from build123d import *
from build123d.topology import SkipClean

# Parameters (mm, degrees)
SKETCH2_R               = 69.85
BOSS_EXTRUDE1_DEPTH     = 4.233333
BOSS_EXTRUDE2_DEPTH     = 38.1
FILLET3_R               = 12.7
FILLET4_R               = 12.7
FILLET5_R               = 12.7
BOSS_EXTRUDE3_DEPTH     = 38.1
CUT_EXTRUDE1_DEPTH      = 108.471653
CUT_EXTRUDE1_DEPTH_BACK = 108.471653
SKETCH5_R               = 4.5085
FILLET6_R               = 12.7


with BuildPart() as part:
    # Sketch2 → Boss-Extrude1 (new body)
    with BuildSketch(Plane(origin=(0, 0, 0), x_dir=(1, 0, 0), z_dir=(0, 1, 0))):
        with Locations(Location((0, 0, 0), (0, 0, 270))):
            Circle(SKETCH2_R)
    extrude(amount=BOSS_EXTRUDE1_DEPTH)

    # Sketch3 → Boss-Extrude2 (add)
    with BuildSketch(Plane(origin=(0, 4.233333, 0), x_dir=(1, 0, 0), z_dir=(0, 1, 0))):
        with BuildLine():
            Line((-16.709043, -54.652817), (-20.422164, -66.797887))
            ThreePointArc((-20.422164, -66.797887), (0, -69.85), (20.422164, -66.797887))
            Line((20.422164, -66.797887), (16.709043, -54.652817))
            ThreePointArc((16.709043, -54.652817), (0, -57.15), (-16.709043, -54.652817))
        make_face()
        with BuildLine():
            ThreePointArc((20.422164, 66.797887), (0, 69.85), (-20.422164, 66.797887))
            Line((-20.422164, 66.797887), (-16.709043, 54.652817))
            ThreePointArc((-16.709043, 54.652817), (0, 57.15), (16.709043, 54.652817))
            Line((16.709043, 54.652817), (20.422164, 66.797887))
        make_face()
    extrude(amount=BOSS_EXTRUDE2_DEPTH)

    # Fillet3
    fillet3_edges = [part.edges().sort_by_distance(p)[0] for p in [
        (-16.709043, 23.283333, -54.652817),
    ]]
    fillet(fillet3_edges, radius=FILLET3_R)

    # Fillet4
    fillet4_edges = [part.edges().sort_by_distance(p)[0] for p in [
        (16.709043, 23.283333, 54.652817),
    ]]
    fillet(fillet4_edges, radius=FILLET4_R)

    # Fillet5
    fillet5_edges = [part.edges().sort_by_distance(p)[0] for p in [
        (-16.709043, 23.283333, 54.652817),
    ]]
    fillet(fillet5_edges, radius=FILLET5_R)

    # Sketch4 → Boss-Extrude3 (add)
    with SkipClean():  # the faces are left unmerged after this step: merging them gives an invalid solid
        with BuildSketch(Plane(origin=(0, 4.233333, 0), x_dir=(1, 0, 0), z_dir=(0, 1, 0))):
            with BuildLine():
                Line((59.670481, 21.718279), (65.63753, 23.890107))
                ThreePointArc((65.63753, 23.890107), (69.85, 0), (65.63753, -23.890107))
                Line((65.63753, -23.890107), (59.670481, -21.718279))
                ThreePointArc((59.670481, -21.718279), (63.5, 0), (59.670481, 21.718279))
            make_face()
        extrude(amount=BOSS_EXTRUDE3_DEPTH)

    # Sketch5 → Cut-Extrude1 (cut, two sides: drawn at the far end of the back side and taken through both)
    with SkipClean():  # the faces are left unmerged after this step: merging them gives an invalid solid
        with BuildSketch(Plane(origin=(0, 42.333333, 0), x_dir=(1, 0, 0), z_dir=(0, 1, 0)).offset(-CUT_EXTRUDE1_DEPTH_BACK)):
            with Locations(Location((0, 63.5, 0), (0, 0, 270))):
                Circle(SKETCH5_R)
            with Locations(Location((0, -63.5, 0), (0, 0, 270))):
                Circle(SKETCH5_R)
        extrude(amount=CUT_EXTRUDE1_DEPTH + CUT_EXTRUDE1_DEPTH_BACK, mode=Mode.SUBTRACT)

    # Fillet6
    fillet6_edges = [part.edges().sort_by_distance(p)[0] for p in [
        (16.709043, 23.283333, -54.652817),
    ]]
    fillet(fillet6_edges, radius=FILLET6_R)


solid = part.part
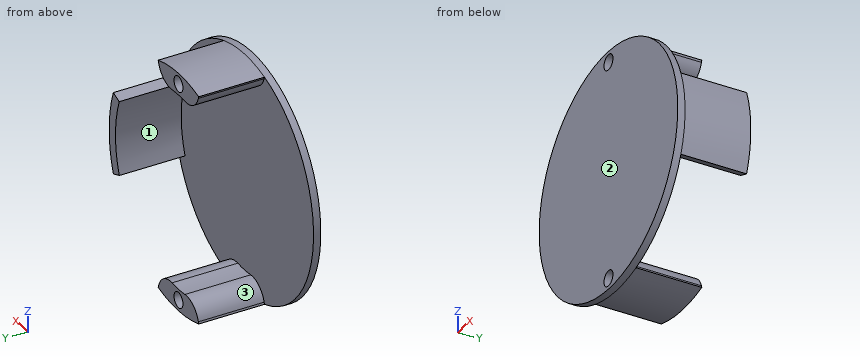
Can you work these out from the model? Positions are in its coordinate system, mm. Face numbers are marked on the shaded views. Coordinates: 2 decimals unless noted, no trailing zeros. Loops run counter-clockwise (first coordinate to the right, second up) from the corner with the lowest first, then second, coordinate; pieces in that order, holes last. Notation, with made-up numbers: M 43.25,-26 L 77.25,-26 A23 cw 77.25,13 Z; hole C -6,73.5 d7. An arc over 180 degrees is marked long. Return JSON: item names as keys, results as strings. Group by question number.
Item 1: Imagine slicing it at D-D (z = 0). Please give me the cut outline in (x, y).
Item 2: Imagine slicing it at B-B (x = 0). Please give me the cut outline in (y, z), and give its area (3 significant figures).
Item 3: If I drill on L1, parallel to Y at x = 0, z = -14; L2, parallel to X at y = 18, z = -63; L3, parallel to X at y = 39, z = -60.5, over which ranges is the centre line in solid material (lowest first)? Write a range as from..to.
Item 4: Imagine slicing it at C-C (z = -63.5). Please give me the cut outline in (x, y).
Item 5: Thinking about a two-plate mould opening in Z: for the marked faces 1, 2 and 3, which applies, released by +Z, released by -Z, zero draft, split by the parting line, or undercut?
Item 6: I'm going to push flat-ended pins straight in: pin 1 Ø1.5 at (y, z) = (17, 9) entering from -X; pin 2 Ø10 at (y, z) = (7, -53.5) entering from -X; pin 3 Ø1.5 at (x, y) = (23, 33.5) entering from -Z; pin 4 Ø12 at (x, z) = (-32.5, -2) entering from +Y. Where does each tip first touch, or does it pass through?
Item 7: Imagine slicing it at A-A (y = 25). Please give me the cut outline in (x, z), and give its area (3 significant figures).
Verdict:
{
 "1": {"outline": "M -69.85,0 L 69.85,0 L 69.85,42.33 L 63.5,42.33 L 63.5,4.23 L -69.85,4.23 Z"},
 "2": {"outline": "M 0,-69.85 L 42.33,-69.85 L 42.33,-68.01 L 0,-68.01 Z; M 0,-58.99 L 42.33,-58.99 L 42.33,-57.15 L 4.23,-57.15 L 4.23,57.15 L 42.33,57.15 L 42.33,58.99 L 0,58.99 Z; M 0,68.01 L 42.33,68.01 L 42.33,69.85 L 0,69.85 Z", "area": "796 mm^2"},
 "3": {"L1": "y = 0..4.23", "L2": "x = -18.91..-4.48, 4.48..18.91", "L3": "x = -17..-3.37, 3.37..17"},
 "4": {"outline": "M -29.1,0 L -4.51,0 L -4.51,42.33 L -19.18,42.33 L -19.18,4.23 L -29.1,4.23 Z; M 4.51,0 L 29.1,0 L 29.1,4.23 L 19.18,4.23 L 19.18,42.33 L 4.51,42.33 Z"},
 "5": {"face 1": "undercut", "face 2": "zero draft", "face 3": "undercut"},
 "6": {"pin 1": "stops at x = 62.75", "pin 2": "stops at x = -49.45", "pin 3": "passes through", "pin 4": "stops at y = 4.23"},
 "7": {"outline": "M -20.42,-66.8 A69.85 ccw 20.42,-66.8 L 20.08,-65.68 A12.7 ccw 6.49,-56.78 A57.15 cw -6.49,-56.78 A12.7 ccw -20.08,-65.68 Z; M -20.42,66.8 L -20.08,65.68 A12.7 ccw -6.49,56.78 A57.15 cw 6.49,56.78 A12.7 ccw 20.08,65.68 L 20.42,66.8 A69.85 ccw Z; M 59.67,-21.72 L 65.64,-23.89 A69.85 ccw 65.64,23.89 L 59.67,21.72 A63.5 cw Z; hole C 0,-63.5 d9.02; hole C 0,63.5 d9.02", "area": "1,020 mm^2"}
}
